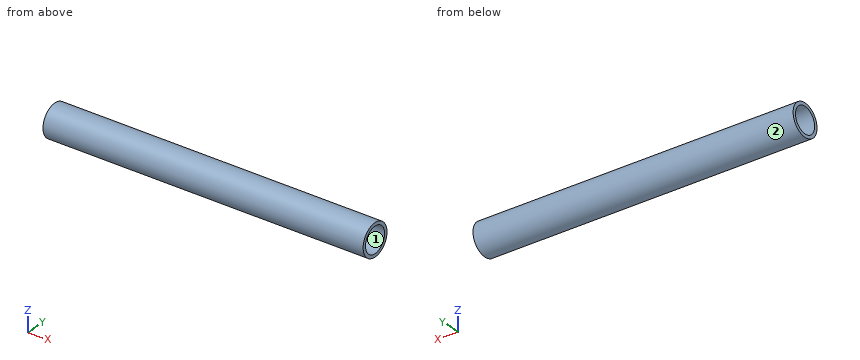
```python
from build123d import *

# Parameters (mm, degrees)
CYLINDER007_R           = 6
CYLINDER007_DEPTH       = 236
CYLINDER007_PITCH_ANGLE = 90
CYLINDER003_R           = 5.5
CYLINDER003_DEPTH       = 150
CYLINDER003_PITCH_ANGLE = 90
CYLINDER_R              = 7.5
CYLINDER_DEPTH          = 150
CYLINDER_PITCH_ANGLE    = 90


with BuildPart() as connector_bore:
    # Cylinder007 → Cylinder007 (new body)
    with BuildSketch(Plane.XY):
        Circle(CYLINDER007_R)
    extrude(amount=CYLINDER007_DEPTH)


with BuildPart() as connector_bore_1:
    # Cylinder007 pitch: moved
    add(connector_bore.part.rotate(Axis((0, 0, 0), (0, 1, 0)), CYLINDER007_PITCH_ANGLE))


with BuildPart() as connector_bore_2:
    # Cylinder007 placement: moved
    add(connector_bore_1.part.moved(Location((-45, 0, 0))))


with BuildPart() as obj1:
    # Cylinder003 → Cylinder003 (new body)
    with BuildSketch(Plane.XY):
        Circle(CYLINDER003_R)
    extrude(amount=CYLINDER003_DEPTH)


with BuildPart() as obj1_1:
    # Cylinder003 pitch: moved
    add(obj1.part.rotate(Axis((0, 0, 0), (0, 1, 0)), CYLINDER003_PITCH_ANGLE))


with BuildPart() as obj1_2:
    # Cylinder003 placement: moved
    add(obj1_1.part)


with BuildPart() as cut006:
    # Cylinder → Cylinder (new body)
    with BuildSketch(Plane.XY):
        Circle(CYLINDER_R)
    extrude(amount=CYLINDER_DEPTH)


with BuildPart() as cut006_1:
    # Cylinder pitch: moved
    add(cut006.part.rotate(Axis((0, 0, 0), (0, 1, 0)), CYLINDER_PITCH_ANGLE))


with BuildPart() as cut006_2:
    # Cylinder placement: moved
    add(cut006_1.part)

    # Cut: cut obj1
    add(obj1_2.part, mode=Mode.SUBTRACT)

    # Cut006: cut connector_bore
    add(connector_bore_2.part, mode=Mode.SUBTRACT)


solid = cut006_2.part
```
The model under review builds one solid part; all positions refer to its coordinate system, in mm. Face numbers are marked on the shaded views. Round coordinates to 2 decimals unless told otherwise and drop trailing zeros. Loops run counter-clockwise (first coordinate to the right, second up) from the corner with the lowest first, then second, coordinate; pieces in that order, holes last.
Item 1: Take a section at C-C (x = 130). Write out the cut boundary in (y, z), then the cut area to 3 significant figures.
Determined:
outline: circle Ø15 at (0, 0); hole circle Ø12 at (0, 0)
area: 63.6 mm2
Item 2: Clearance check with flat-ended pins moving along their axes: pin 1 Ø6 at (y, z) = (-5, -6) entering from +X; pin 2 Ø1.5 at (x, y) = (56, 3.5) entering from -Z; pin 3 Ø3 at (x, y) = (25.5, 4.5) entering from -Z. State where each tip first meets the part, or that it passes through.
Determined:
pin 1: stops at x = 150
pin 2: stops at z = -6.98
pin 3: stops at z = -6.87
Item 3: Take a section at A-A (y = 0). Write out the cut boundary in (x, z).
Determined:
outline: (0, -7.5) - (150, -7.5) - (150, -6) - (0, -6) - close; (0, 6) - (150, 6) - (150, 7.5) - (0, 7.5) - close
Item 4: For line 1 (Y direction, x = 103, z = -0.5); line 2 (Z direction, x = 55.5, y = 2); line 3 (Z direction, x = 14.5, y = -2.5), list the stretches that pass through material, from the lowest coordinate up.
Determined:
line 1: y = -7.48 to -5.98, 5.98 to 7.48
line 2: z = -7.23 to -5.66, 5.66 to 7.23
line 3: z = -7.07 to -5.45, 5.45 to 7.07
Item 5: Mouldability with a two-part tool opening along Z and no side actions: class the marked faces 1 and 2 as released by +Z, released by -Z, zero draft, split by the parting line, or undercut.
Determined:
face 1: undercut
face 2: split by the parting line
